Read the model definition and answer for the solid it produces. Units are mm, in the model's axes. Face numbers are marked on the shaded views. A direction names the side the tool comes from. Round coordinates to 2 decimals unless told otherwise and drop trailing zeros. Write each loop counter-clockwise with the first axis right and the second up, starting at its lowest first coordinate (ties: lowest second). Pieces come first, ordered by that corner, then holes. Notation, with made-up numbers: (-27.75, -5.75) -> (31.25, -5.75) arc R26 ccw to (31.25, 12.25) -> close; hole circle Ø7 at (47.5, -21). An arc over 180 degrees is marked (long way). Return JSON: item names as keys, results as strings. Group by question number.
(1) A cutting plane is placed at A-A on x = 110. Give the vertices of the cut face in (y, z), then the cut area to 3 significant figures.
(2) A cutting plane is placed at B-B on y = 10. Give the vertices of the cut face in (x, z), then the cut area to 3 significant figures.
(3) For the marked faces 5 and 6, determine the directions among +Z, -Z, +X, -X, +Y, -Y from which every point of the face is accessible in a straight line to the end or side of a thin tool.
(4) Given pin 1 (9 mm diameter, centred on x = 110, y = 10, fed in from +Z); pin 2 (11.5 mm diameter, centred on x = 30, y = 10, fed in from -Z); pin 3 (18 mm diameter, centred on x = 63.5, z = -16.5, fed in from +Y); pin 4 (2 mm diameter, centred on x = 67.5, z = -0.5, fed in from +Y), each flat-ended and moving along its own axis, determine where each tip first touches the part or whether it passes through.
(5) Straight lines are drawn through the part: line 1 (Z direction, x = 35, y = 14); line 2 (Y direction, x = 56.5, z = -4); line 3 (Y direction, x = 110, z = -38.8). For each, find the intervals that lie inside material, in ascending order.
(6) A cutting plane is placed at C-C on y = 18. Give the vertices of the cut face in (x, z), then the cut area to 3 significant figures.
(7) The mould has two halves that part along Z. Classify the marked faces 1, 2, 3 and 4: released by +Z, released by -Z, zero draft, split by the parting line, or undercut.
(8) A cutting plane is placed at D-D on z = -22.5. Give the vertices of the cut face in (x, y), then the cut area to 3 significant figures.
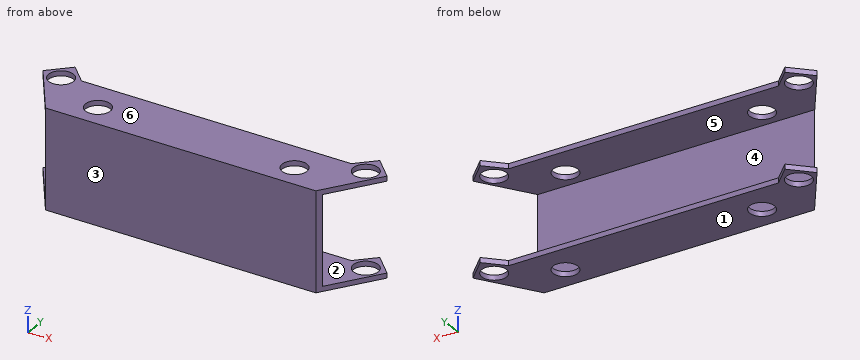
```python
from build123d import *

# Parameters (mm, degrees)
SKETCH1_W           = 140
SKETCH1_H           = 40
BOSS_EXTRUDE1_DEPTH = 30
SKETCH2_W           = 36
SKETCH2_H           = 28
CUT_EXTRUDE1_DEPTH  = 149.660687473
CUT_EXTRUDE2_DEPTH  = 149.660687473
CUT_EXTRUDE3_DEPTH  = 149.660687473
SKETCH6_R           = 5
CUT_EXTRUDE6_DEPTH  = 149.660687473


with BuildPart() as part:
    # Sketch1 → Boss-Extrude1 (new body)
    with BuildSketch(Plane(origin=(0, 0, 0), x_dir=(1, 0, 0), z_dir=(0, 1, 0))):
        with Locations((70, 20)):
            Rectangle(SKETCH1_W, SKETCH1_H)
    extrude(amount=BOSS_EXTRUDE1_DEPTH)

    # Sketch2 → Cut-Extrude1 (cut, through all)
    with BuildSketch(Plane(origin=(140, 0, 0), x_dir=(0, 0, -1), z_dir=(1, 0, 0))):
        with Locations((20, 16)):
            Rectangle(SKETCH2_W, SKETCH2_H)
    extrude(amount=-CUT_EXTRUDE1_DEPTH, mode=Mode.SUBTRACT)

    # Sketch3 → Cut-Extrude2 (cut, through all)
    with BuildSketch(Plane.XY):
        Polygon((0, 0), (15, 0), (0, 22), align=None)
        Polygon((140, 22), (125, 0), (140, 0), align=None)
    extrude(amount=-CUT_EXTRUDE2_DEPTH, mode=Mode.SUBTRACT)

    # Sketch5 → Cut-Extrude3 (cut, through all)
    with BuildSketch(Plane.XY):
        Polygon((0, 30), (0, 22), (8, 30), align=None)
        Polygon((140, 30), (132, 30), (140, 22), align=None)
    extrude(amount=-CUT_EXTRUDE3_DEPTH, mode=Mode.SUBTRACT)

    # Sketch6 → Cut-Extrude6 (cut, through all)
    with BuildSketch(Plane.XY):
        Polygon((70, 30), (8, 30), (15.107268728, 22.892731272), (70, 22.892731272), align=None)
        Polygon((132, 30), (70, 30), (70, 22.892731272), (124.892731272, 22.892731272), align=None)
        with Locations((132, 21)):
            Circle(SKETCH6_R)
        with Locations((110, 10)):
            Circle(SKETCH6_R)
        with Locations((30, 10)):
            Circle(SKETCH6_R)
        with Locations((8, 21)):
            Circle(SKETCH6_R)
    extrude(amount=-CUT_EXTRUDE6_DEPTH, mode=Mode.SUBTRACT)


solid = part.part
```
Checks:
{
 "1": {"outline": "(0, -40) -> (5, -40) -> (5, -38) -> (2, -38) -> (2, -2) -> (5, -2) -> (5, 0) -> (0, 0) -> close; (15, -40) -> (22.89, -40) -> (22.89, -38) -> (15, -38) -> close; (15, -2) -> (22.89, -2) -> (22.89, 0) -> (15, 0) -> close", "area": "124 mm^2"},
 "2": {"outline": "(8.18, -40) -> (25, -40) -> (25, -38) -> (8.18, -38) -> close; (8.18, -2) -> (25, -2) -> (25, 0) -> (8.18, 0) -> close; (35, -40) -> (105, -40) -> (105, -38) -> (35, -38) -> close; (35, -2) -> (105, -2) -> (105, 0) -> (35, 0) -> close; (115, -40) -> (131.82, -40) -> (131.82, -38) -> (115, -38) -> close; (115, -2) -> (131.82, -2) -> (131.82, 0) -> (115, 0) -> close", "area": "415 mm^2"},
 "3": {"face 5": "+X, -X, +Y", "face 6": "+Z, +X, -X, +Y, -Y"},
 "4": {"pin 1": "passes through", "pin 2": "stops at z = -40", "pin 3": "stops at y = 2", "pin 4": "stops at y = 22.89"},
 "5": {"line 1": "z = -40 to -38, -2 to 0", "line 2": "y = 0 to 2", "line 3": "y = 0 to 5, 15 to 22.89"},
 "6": {"outline": "(2.73, -40) -> (4, -40) -> (4, -38) -> (2.73, -38) -> close; (2.73, -2) -> (4, -2) -> (4, 0) -> (2.73, 0) -> close; (12, -40) -> (128, -40) -> (128, -38) -> (12, -38) -> close; (12, -2) -> (128, -2) -> (128, 0) -> (12, 0) -> close; (136, -40) -> (137.27, -40) -> (137.27, -38) -> (136, -38) -> close; (136, -2) -> (137.27, -2) -> (137.27, 0) -> (136, 0) -> close", "area": "474 mm^2"},
 "7": {"face 1": "released by -Z", "face 2": "undercut", "face 3": "zero draft", "face 4": "undercut"},
 "8": {"outline": "(13.64, 2) -> (15, 0) -> (125, 0) -> (126.36, 2) -> close", "area": "223 mm^2"}
}
